Autodesk Inventor part; units mm, degrees
ref_plane "YZ Plane" through (0, 0, 0) normal (1, 0, 0) x (0, 1, 0)
ref_plane "XZ Plane" through (0, 0, 0) normal (0, 1, 0) x (-1, 0, 0)
ref_plane "XY Plane" through (0, 0, 0) normal (0, 0, 1) x (1, 0, 0)
sketch "Boceto1" plane through (0, 0, 0) normal (0, 1, 0) x (-1, 0, 0)
  line L0 (0, 0) -> (262.4667, 0) construction
  line L1 (262.4667, 0) -> (262.4667, -371.2633) construction
  line L2 (262.4667, -371.2633) -> (0, -371.2633) construction
  line L3 (0, -371.2633) -> (0, 0) construction
  line L4 (167.9771, -4.7349) -> (167.9771, -13.5349)
  line L5 (167.9771, -13.5349) -> (2.3545, -13.5349)
  line L6 (2.3545, -13.5349) -> (2.3545, -4.7349)
  line L7 (2.3545, -4.7349) -> (167.9771, -4.7349)
  line L8 (143.5689, -182.4039) -> (2.3545, -182.4039)
  line L9 (2.3545, -182.4039) -> (2.3545, -173.6039)
  line L10 (2.3545, -173.6039) -> (167.9771, -173.6039)
  line L11 (167.9771, -173.6039) -> (167.9771, -182.4039)
  circle A0 centre (156.1475, -9.1349) radius 2
  circle A1 centre (131.2333, -9.1349) radius 2
  circle A2 centre (12.066, -9.1349) radius 2
  line L12 (167.9771, -173.6039) -> (167.9771, -182.4039)
  line L13 (167.9771, -182.4039) -> (2.3545, -182.4039)
  line L14 (2.3545, -182.4039) -> (2.3545, -173.6039)
  line L15 (2.3545, -173.6039) -> (167.9771, -173.6039)
  circle A3 centre (131.2333, -178.0039) radius 2
  circle A4 centre (12.066, -178.0039) radius 2
  line L16 (167.9771, -13.5349) -> (167.9771, -182.4039)
  line L17 (2.3545, -13.4261) -> (2.3545, -174.0455)
  line L18 (11.1545, -13.4261) -> (11.1545, -174.0455)
  line L19 (159.1771, -13.5349) -> (159.1771, -182.4039)
  line L20 (26.8486, -4.7349) -> (26.8486, -49.7349)
  line L21 (26.8486, -49.7349) -> (2.3545, -49.7349)
  line L22 (35.6486, -4.7349) -> (35.6486, -173.6039)
  line L23 (35.6486, -58.5349) -> (2.3545, -58.5349)
  line L24 (2.3545, -59.0349) -> (36.1486, -59.0349)
  line L25 (36.1486, -173.6039) -> (36.1486, -4.7349)
  line L26 (2.3545, -67.8349) -> (44.9486, -67.8349)
  line L27 (44.9486, -67.8349) -> (44.9486, -4.7349)
  line L28 (26.8486, -49.7349) -> (26.8486, -173.6039)
  line L29 (19.9545, -13.4261) -> (19.9545, -174.0455)
  line L30 (9.3545, -13.4261) -> (9.3545, -174.0455)
  point P0 (11.1545, -173.6039)
  point P1 (11.1545, -13.5349)
  point P2 (159.1771, -173.6039)
  point P3 (11.1545, -58.5349)
  point P4 (35.6486, -13.5349)
  point P5 (11.1545, -67.8349)
  point P6 (26.8486, -67.8349)
  point P7 (36.1486, -67.8349)
  dimension "d2" = 8.8
  dimension "d3" = 8.8
  dimension "d5" = 8.8
  dimension "d6" = 8.8
  dimension "d8" = 4
  dimension "d9" = 4
  dimension "d10" = 4
  dimension "d11" = 8.8
  dimension "d12" = 8.8
  dimension "d14" = 4
  dimension "d15" = 4
  dimension "d21" = 8.8
  dimension "d22" = 8.8
  dimension "d26" = 45
  dimension "d27" = 8.8
  dimension "d53" = 0.5
  dimension "d54" = 8.8
  dimension "d59" = 8.8
  dimension "d60" = 7
extrude "Extrusión1" add sketch "Boceto1" along normal blind 3 contours L4 L5 L27 L7 | L16 L10 L19 L5 | L27 L5 L25 L7 | L11 L13 L19 L10 | L25 L5 L22 L7 | L19 L13 L8 L9 L10 | L22 L5 L20 L7 | L22 L23 L28 L20 L5 | L10 L28 L26 L22 | L22 L24 L28 L23 | L22 L26 L28 L24
sketch "Boceto2" plane through (0, 3, 0) normal (0, 1, 0) x (1, 0, 0)
  line L0 (-2.3545, 182.4039) -> (-167.9771, 182.4039)
  line L1 (-167.9771, 182.4039) -> (-167.9771, 4.7349)
  line L2 (-167.9771, 4.7349) -> (-26.8486, 4.7349)
  circle A0 centre (-12.066, 178.0039) radius 2
  circle A1 centre (-131.2333, 178.0039) radius 2
  circle A2 centre (-156.1475, 9.1349) radius 2
  circle A3 centre (-131.2333, 9.1349) radius 2
  line L3 (-11.1545, 173.6039) -> (-11.1545, 67.8349)
  line L4 (-35.6486, 13.5349) -> (-159.1771, 13.5349)
  line L5 (-159.1771, 13.5349) -> (-159.1771, 173.6039)
  line L6 (-159.1771, 173.6039) -> (-35.6486, 173.6039)
  line L7 (-131.2333, 9.1349) -> (-119.9333, 9.1349)
  line L8 (-119.9333, 9.1349) -> (-119.9333, 13.5349)
  line L9 (-119.9333, 4.7349) -> (-119.9333, 9.1349)
  line L10 (-167.9771, 4.7349) -> (-26.8486, 4.7349)
  line L11 (-26.8486, 4.7349) -> (-26.8486, 173.6039)
  line L12 (-26.8486, 49.7349) -> (-2.3545, 49.7349)
  line L13 (-2.3545, 173.6039) -> (-2.3545, 182.4039)
  line L14 (-11.1545, 58.5349) -> (-35.6486, 58.5349)
  line L15 (-35.6486, 173.6039) -> (-35.6486, 13.5349)
  circle A4 centre (-36.9802, 178.0039) radius 2
  circle A5 centre (-156.1475, 178.0039) radius 2
  circle A6 centre (-156.1475, 9.1349) radius 2
  line L16 (-156.1475, 9.1349) -> (-144.8475, 9.1349)
  line L17 (-144.8475, 9.1349) -> (-144.8475, 13.5349)
  line L18 (-144.8475, 4.7349) -> (-144.8475, 9.1349)
  line L19 (-36.9802, 178.0039) -> (-36.9802, 9.1349)
  line L20 (-36.9802, 178.0039) -> (131.8887, 178.0039) construction
  circle A7 centre (-36.9802, 9.1349) radius 2
  point P0 (0, 0)
  point P1 (-2.3545, 4.7349)
  point P2 (-26.8486, 59.0349)
  point P3 (-2.3545, 59.0349)
  point P4 (-35.6486, 67.8349)
  dimension "d25" = 11.3
  dimension "d29" = 11.3
  dimension "d30" = 90
  dimension "d31" = 4
hole "Agujero1" at (-36.9802, 3, -9.1349) at (-36.9802, 3, -178.0039) at (-156.1475, 3, -178.0039) direction (0, -1, 0) diameter 4 end through all
sketch "Boceto3" plane through (0, 0, 0) normal (0, -1, 0) x (1, 0, 0)
  circle A0 centre (-156.1475, -178.0039) radius 2
  circle A1 centre (-36.9802, -178.0039) radius 2
  circle A2 centre (-36.9802, -9.1349) radius 2
  line L0 (-167.9771, -182.4039) -> (-167.9771, -4.7349)
  line L1 (-2.3545, -182.4039) -> (-167.9771, -182.4039)
  line L2 (-2.3545, -173.6039) -> (-2.3545, -182.4039)
  line L3 (-26.8486, -4.7349) -> (-26.8486, -173.6039)
  line L4 (-167.9771, -4.7349) -> (-26.8486, -4.7349)
  circle A3 centre (-156.1475, -9.1349) radius 2
  circle A4 centre (-131.2333, -9.1349) radius 2
  line L5 (-159.1771, -173.6039) -> (-11.1545, -173.6039)
  line L6 (-159.1771, -13.5349) -> (-159.1771, -173.6039)
  line L7 (-35.6486, -13.5349) -> (-159.1771, -13.5349)
  line L8 (-35.6486, -173.6039) -> (-35.6486, -13.5349)
  circle A5 centre (-131.2333, -178.0039) radius 2
  circle A6 centre (-12.066, -178.0039) radius 2
  line L9 (-36.9802, -9.1349) -> (-46.9802, -9.1349)
  line L10 (-46.9802, -9.1349) -> (-46.9802, -2.3988)
  line L11 (-46.9802, -2.3988) -> (-46.9802, -182.4039)
  line L12 (-131.2333, -9.1349) -> (-121.2333, -9.1349)
  line L13 (-121.2333, -9.1349) -> (-121.2333, 4.8486)
  line L14 (-121.2333, 4.8486) -> (-121.2333, -182.4039)
  line L15 (-159.1771, -173.6039) -> (-167.9771, -173.6039)
  line L16 (-159.1771, -13.5349) -> (-167.9771, -13.5349)
  line L17 (-35.932, -13.5349) -> (-26.8486, -13.5349)
  line L18 (-11.1545, -173.6039) -> (-2.3545, -173.6039)
  line L19 (-2.3545, -172.6039) -> (-11.1545, -172.6039)
  line L20 (-11.1545, -172.6039) -> (-159.1771, -172.6039)
  line L21 (-159.1771, -172.6039) -> (-167.9771, -172.6039)
  line L22 (-35.932, -14.5349) -> (-26.8486, -14.5349)
  line L23 (-159.1771, -14.5349) -> (-167.9771, -14.5349)
  circle A7 centre (-156.1475, -178.0039) radius 2
  circle A8 centre (-36.9802, -178.0039) radius 2
  circle A9 centre (-36.9802, -9.1349) radius 2
  line L24 (-167.9771, -182.4039) -> (-167.9771, -4.7349)
  line L25 (-2.3545, -182.4039) -> (-167.9771, -182.4039)
  line L26 (-2.3545, -173.6039) -> (-2.3545, -182.4039)
  line L27 (-26.8486, -4.7349) -> (-26.8486, -173.6039)
  line L28 (-167.9771, -4.7349) -> (-26.8486, -4.7349)
  circle A10 centre (-12.066, -178.0039) radius 2
  circle A11 centre (-131.2333, -178.0039) radius 2
  circle A12 centre (-131.2333, -9.1349) radius 2
  circle A13 centre (-156.1475, -9.1349) radius 2
  line L29 (-26.8486, -173.6039) -> (-2.3545, -173.6039)
  line L30 (-159.1771, -13.5349) -> (-159.1771, -173.6039)
  line L31 (-35.6486, -13.5349) -> (-159.1771, -13.5349)
  line L32 (-35.6486, -173.6039) -> (-35.6486, -13.5349)
  line L33 (-159.1771, -173.6039) -> (-35.6486, -173.6039)
  circle A14 centre (-156.1475, -178.0039) radius 2
  circle A15 centre (-36.9802, -178.0039) radius 2
  circle A16 centre (-36.9802, -9.1349) radius 2
  line L34 (-167.9771, -182.4039) -> (-167.9771, -4.7349)
  line L35 (-2.3545, -182.4039) -> (-167.9771, -182.4039)
  line L36 (-2.3545, -173.6039) -> (-2.3545, -182.4039)
  line L37 (-26.8486, -173.6039) -> (-2.3545, -173.6039)
  line L38 (-26.8486, -4.7349) -> (-26.8486, -173.6039)
  line L39 (-167.9771, -4.7349) -> (-26.8486, -4.7349)
  circle A17 centre (-12.066, -178.0039) radius 2
  circle A18 centre (-131.2333, -178.0039) radius 2
  circle A19 centre (-131.2333, -9.1349) radius 2
  circle A20 centre (-156.1475, -9.1349) radius 2
  line L40 (-159.1771, -173.6039) -> (-35.6486, -173.6039)
  line L41 (-159.1771, -13.5349) -> (-159.1771, -173.6039)
  line L42 (-35.6486, -13.5349) -> (-159.1771, -13.5349)
  line L43 (-35.6486, -173.6039) -> (-35.6486, -13.5349)
  point P0 (0, 0)
  point P1 (-35.6486, -58.5349)
  point P2 (-35.6486, -14.5349)
  point P3 (-121.2333, -173.6039)
  point P4 (-46.9802, -173.6039)
  point P5 (-121.2333, -13.5349)
  point P6 (-46.9802, -13.5349)
  point P7 (-46.9802, -4.7349)
  point P8 (-121.2333, -4.7349)
  point P9 (-26.8486, -59.0349)
  point P10 (-35.6486, -67.8349)
  point P11 (-35.6486, -172.6039)
  point P12 (-26.8486, -172.6039)
  dimension "d39" = 10
  dimension "d40" = 10
  dimension "d41" = 1
  dimension "d42" = 1
  dimension "d43" = 1
extrude "Extrusión2" add sketch "Boceto3" along normal blind 5 contours L11 L7 L14 L13 L4 L10 | L11 L1 L14 L5 | L8 L22 L3 L20 | L6 L21 L0 L23
properties part number "Base PCB"
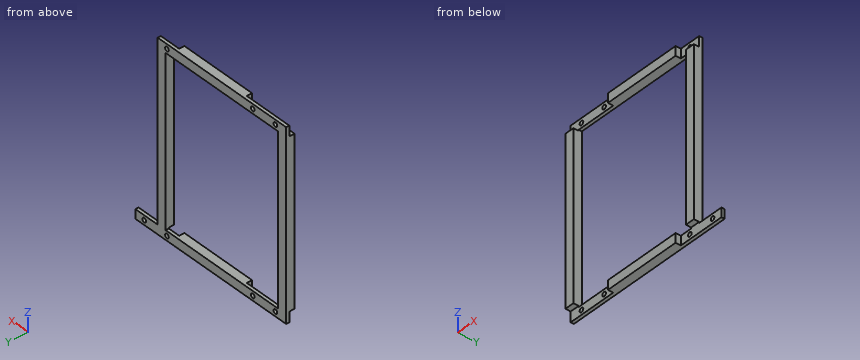
Model file for the job. Use its own axes, mm. Coordinates: 2 decimals unless noted, no trailing zeros. Order: outer loops, then holes, each group sorted by start corner. A loop starts at its lowest first (then second) coordinate and runs counter-clockwise, first axis right, second up. Notation, with made-up numbers: M 51,21.5 L 64,21.5 A8 cw 64,30.5 Z; hole C -15.75,-7 d11. An arc over 180 degrees is marked long. Answer as CSV lines item,"result".
(1) Band-saw the part on C-C, the plane y = -1.25. List the corners of the cut face in (x, z).
Geometry says:
outline,"M -167.98,-172.6 L -159.18,-172.6 L -159.18,-14.53 L -167.98,-14.53 Z; M -121.23,-182.4 L -46.98,-182.4 L -46.98,-173.6 L -121.23,-173.6 Z; M -121.23,-13.53 L -46.98,-13.53 L -46.98,-4.73 L -121.23,-4.73 Z; M -35.65,-172.6 L -26.85,-172.6 L -26.85,-14.53 L -35.65,-14.53 Z"
(2) Band-saw the part on D-D, the plane x = -31.5. List the corners of the cut face in (y, z), then the cut area to 3 significant figures.
Geometry says:
outline,"M -5,-172.6 L 0,-172.6 L 0,-182.4 L 3,-182.4 L 3,-4.73 L 0,-4.73 L 0,-14.53 L -5,-14.53 Z"
area,"1,320 mm2"
(3) Flat gauge pins, fed straight in: pin 1 (3 mm diameter, centred on x = -137, z = -8, fed in from -Y); pin 2 (2.5 mm diameter, centred on y = -2, z = -9.5, fed in from -X); pin 3 (2.5 mm diameter, centred on y = -3.5, z = -179, fed in from +X). Where does each tip first touch, or does it go through?
Geometry says:
pin 1,"stops at y = 0"
pin 2,"stops at x = -121.23"
pin 3,"stops at x = -46.98"
(4) Band-saw the part on B-B, the plane z = -26. List the corners of the cut face in (x, y).
Geometry says:
outline,"M -167.98,-5 L -159.18,-5 L -159.18,3 L -167.98,3 Z; M -35.65,-5 L -26.85,-5 L -26.85,3 L -35.65,3 Z"
(5) Band-saw the part on A-A, the plane x = -149. List the corners of the cut face in (y, z), then the cut area to 3 significant figures.
Geometry says:
outline,"M 0,-182.4 L 3,-182.4 L 3,-173.6 L 0,-173.6 Z; M 0,-13.53 L 3,-13.53 L 3,-4.73 L 0,-4.73 Z"
area,"52.8 mm2"
(6) Wall check: line 1 along Z through (x, y) = (-115.5, -2); line 2 along X through (y, z) = (-2, -88); line 3 along Z through (x, y) = (-25.5, 1). Give the ranges that are in metal, low to high.
Geometry says:
line 1,"z = -182.4 to -173.6, -13.53 to -4.73"
line 2,"x = -167.98 to -159.18, -35.65 to -26.85"
line 3,"z = -182.4 to -173.6"
